Model file for the job. Use its own axes, mm. A direction names the side the tool comes from. Round coordinates to 2 decimals unless told otherwise and drop trailing zeros. Write each loop counter-clockwise with the first axis right and the second up, starting at its lowest first coordinate (ties: lowest second). Pieces come first, ordered by that corner, then holes. Notation, with made-up numbers: (70, -15.5) - (82, -15.5) arc R17 ccw to (82, 15.5) - close; hole circle Ø5 at (42.5, 79). An arc over 180 degrees is marked (long way). One line per item, written item: value.
from build123d import *

# Parameters (mm, degrees)
SKETCH_1_W          = 40
SKETCH_1_H          = 20
EXTRUDE_1_DEPTH     = 40.5
SKETCH_2_W          = 7.25
SKETCH_2_H          = 20
EXTRUDE_2_DEPTH     = 3
SKETCH_3_R          = 2
CUT_EXTRUDE_1_DEPTH = 5
SKETCH_4_R          = 3
EXTRUDE_3_DEPTH     = 3


with BuildPart() as part:
    # 草图1 → 凸台-拉伸1 (new body)
    with BuildSketch(Plane.XY):
        Rectangle(SKETCH_1_W, SKETCH_1_H)
    extrude(amount=EXTRUDE_1_DEPTH)

    # 草图2 → 凸台-拉伸2 (add)
    with BuildSketch(Plane(origin=(0, 0, 27.8), x_dir=(-1, 0, 0), z_dir=(0, 0, -1))):
        with Locations((-23.625, 0)):
            Rectangle(SKETCH_2_W, SKETCH_2_H)
        with Locations((23.625, 0)):
            Rectangle(SKETCH_2_W, SKETCH_2_H)
    extrude(amount=-EXTRUDE_2_DEPTH)

    # 草图3 → 切除-拉伸1 (cut)
    with BuildSketch(Plane.XY.offset(30.8)):
        with Locations((-24.75, 5)):
            Circle(SKETCH_3_R)
        with Locations((-24.75, -5)):
            Circle(SKETCH_3_R)
        with Locations(Location((24.75, -5, 0), (0, 0, 180))):
            Circle(SKETCH_3_R)
        with Locations(Location((24.75, 5, 0), (0, 0, 180))):
            Circle(SKETCH_3_R)
    extrude(amount=-CUT_EXTRUDE_1_DEPTH, mode=Mode.SUBTRACT)

    # 草图4 → 凸台-拉伸3 (add)
    with BuildSketch(Plane.XY.offset(40.5)):
        with Locations((10.1, 0)):
            Circle(SKETCH_4_R)
    extrude(amount=EXTRUDE_3_DEPTH)


solid = part.part
1. Band-saw the part on D-D on y = 0. Write the cut outline in (x, z), plus the area to 3 significant figures.
Report:
outline: (-27.25, 27.8) - (-20, 27.8) - (-20, 0) - (20, 0) - (20, 27.8) - (27.25, 27.8) - (27.25, 30.8) - (20, 30.8) - (20, 40.5) - (13.1, 40.5) - (13.1, 43.5) - (7.1, 43.5) - (7.1, 40.5) - (-20, 40.5) - (-20, 30.8) - (-27.25, 30.8) - close
area: 1,680 mm²
2. Band-saw the part on C-C on x = 8.5. Write the cut outline in (y, z).
Report:
outline: (-10, 0) - (10, 0) - (10, 40.5) - (2.54, 40.5) - (2.54, 43.5) - (-2.54, 43.5) - (-2.54, 40.5) - (-10, 40.5) - close
3. Band-saw the part on A-A on x = 24.75. Write the cut outline in (y, z).
Report:
outline: (-10, 27.8) - (-7, 27.8) - (-7, 30.8) - (-10, 30.8) - close; (-3, 27.8) - (3, 27.8) - (3, 30.8) - (-3, 30.8) - close; (7, 27.8) - (10, 27.8) - (10, 30.8) - (7, 30.8) - close
4. Band-saw the part on B-B on y = 5. Write the cut outline in (x, z), plus the area to 3 significant figures.
Report:
outline: (-27.25, 27.8) - (-26.75, 27.8) - (-26.75, 30.8) - (-27.25, 30.8) - close; (-22.75, 27.8) - (-20, 27.8) - (-20, 0) - (20, 0) - (20, 27.8) - (22.75, 27.8) - (22.75, 30.8) - (20, 30.8) - (20, 40.5) - (-20, 40.5) - (-20, 30.8) - (-22.75, 30.8) - close; (26.75, 27.8) - (27.25, 27.8) - (27.25, 30.8) - (26.75, 30.8) - close
area: 1,640 mm²
5. Mould opens along Y. For faces 1 (the face through (27.25, 0, 29)), 2 (the face through (0, 10, 20)), 3 (the face through (-26.337, -6.217, 29.321)) say: released by +Y, released by -Y, zero draft, split by the parting line, or undercut.
Report:
face 1: zero draft
face 2: released by +Y
face 3: undercut
6. Wall check: probe 1 along Y at (x, z) = (24.75, 30.2); probe 2 along Y at (x, z) = (-24, 30); probe 3 along X at (y, z) = (3.75, 9.5). Give the ranges that are in metal, low to high. Write a range as [from, to].
Report:
probe 1: [-10, -7], [-3, 3], [7, 10]
probe 2: [-10, -6.85], [-3.15, 3.15], [6.85, 10]
probe 3: [-20, 20]
7. Drop flat-ended pins along their axis: pin 1 (6 mm diameter, centred on x = 23.5, y = 2, fed in from -Z); pin 2 (5 mm diameter, centred on x = -21, y = -7, fed in from -Z); pin 3 (3 mm diameter, centred on x = 10, y = -5.5, fed in from +Z); pin 4 (1 mm diameter, centred on y = -2.5, z = 7.5, fed in from -X). Give the stop position or say it passes through.
Report:
pin 1: z = 27.8
pin 2: z = 0
pin 3: z = 40.5
pin 4: x = -20
8. Tool access for faces 4 (the face through (-20, 0, 14)), 5 (the face through (20, 0, 36)), 6 (the face through (-20, 0, 36)), 7 (the face through (20, 0, 14)): list every direction of +Z, -Z, +X, -X, +Y, -Y with a clear straight run to the whole face (end or side of a thin tool).
Report:
face 4: -Z, -X, +Y, -Y
face 5: +Z, +X, +Y, -Y
face 6: +Z, -X, +Y, -Y
face 7: -Z, +X, +Y, -Y
